from build123d import *

# Parameters (mm, degrees)
SKETCH1_W            = 174
SKETCH1_H            = 65
BOSS_EXTRUDE1_DEPTH  = 5
SKETCH2_W            = 174
SKETCH2_H            = 65
SKETCH2_W_2          = 168
SKETCH2_H_2          = 59
BOSS_EXTRUDE2_DEPTH  = 23
CUT_EXTRUDE2_DEPTH   = 23
SKETCH4_R            = 1.25
CUT_EXTRUDE3_DEPTH   = 4
LPATTERN2_COUNT      = 2
LPATTERN2_PITCH      = 62
LPATTERN2_COUNT_DIR2 = 2
LPATTERN2_PITCH_DIR2 = 171
CUT_EXTRUDE4_DEPTH   = 10


with BuildPart() as part:
    # Sketch1 → Boss-Extrude1 (new body)
    with BuildSketch(Plane(origin=(0, 0, 0), x_dir=(1, 0, 0), z_dir=(0, 1, 0))):
        with Locations((87, 32.5)):
            Rectangle(SKETCH1_W, SKETCH1_H)
    extrude(amount=BOSS_EXTRUDE1_DEPTH)

    # Sketch2 → Boss-Extrude2 (add)
    with BuildSketch(Plane(origin=(0, 5, 0), x_dir=(1, 0, 0), z_dir=(0, 1, 0))):
        with Locations((87, 32.5)):
            Rectangle(SKETCH2_W, SKETCH2_H)
        with Locations((87, 32.5)):
            Rectangle(SKETCH2_W_2, SKETCH2_H_2, mode=Mode.SUBTRACT)
    extrude(amount=BOSS_EXTRUDE2_DEPTH)

    # Sketch3 → Cut-Extrude2 (cut)
    with BuildSketch(Plane(origin=(174, 0, 0), x_dir=(0, 0, -1), z_dir=(1, 0, 0))):
        with BuildLine():
            Line((29.5, 22), (37.5, 22))
            ThreePointArc((37.5, 22), (39.25, 20.25), (37.5, 18.5))
            Line((37.5, 18.5), (29.5, 18.5))
            ThreePointArc((29.5, 18.5), (27.75, 20.25), (29.5, 22))
        make_face()
    extrude(amount=-CUT_EXTRUDE2_DEPTH, mode=Mode.SUBTRACT)

    # Sketch4 → Cut-Extrude3 (cut)
    with BuildSketch(Plane(origin=(0, 28, 0), x_dir=(1, 0, 0), z_dir=(0, 1, 0))):
        with Locations((1.5, 1.5)):
            Circle(SKETCH4_R)
    cut_extrude3 = extrude(amount=-CUT_EXTRUDE3_DEPTH, mode=Mode.SUBTRACT)

    # LPattern2: Cut-Extrude3 2 × 2
    with Locations(*[(j * LPATTERN2_PITCH_DIR2, 0, -i * LPATTERN2_PITCH) for i in range(LPATTERN2_COUNT) for j in range(LPATTERN2_COUNT_DIR2) if (i, j) != (0, 0)]):
        add(cut_extrude3, mode=Mode.SUBTRACT)

    # Sketch5 → Cut-Extrude4 (cut)
    with BuildSketch(Plane.XY):
        with BuildLine():
            Line((128, 15.55), (118, 15.55))
            ThreePointArc((118, 15.55), (115.5, 18.05), (118, 20.55))
            Line((118, 20.55), (128, 20.55))
            ThreePointArc((128, 20.55), (130.5, 18.05), (128, 15.55))
        make_face()
    extrude(amount=-CUT_EXTRUDE4_DEPTH, mode=Mode.SUBTRACT)


solid = part.part
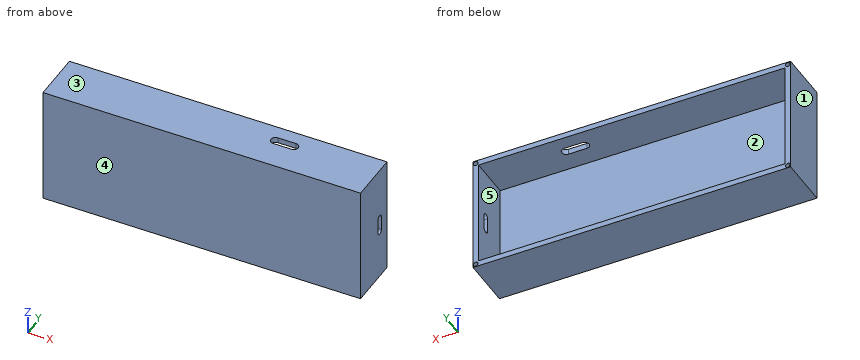
Verification items for the finished model (mm, model axes). Face numbers are marked on the shaded views. A direction names the side the tool comes from. Give positions to 0.01 mm unless a question says otherwise; leave off trailing zeros. Order: outer loops, then holes, each group sorted by start corner. A loop starts at its lowest first (then second) coordinate and runs counter-clockwise, first axis right, second up. Notation, with made-up numbers: M 50,9.25 L 74,9.25 A26 cw 74,24.25 Z; hole C 84,-4.5 d4. An arc over 180 degrees is marked long. Use one line per item in the form item = value. Start each with the question number.
Q1. Go/stop test with flat-tipped pins: pin 1 Ø2 at (x, z) = (172.5, -1.5) entering from +Y; pin 2 Ø1 at (x, z) = (31, -51.5) entering from +Y. Record where each tip stops, or that it passes through.
Q2. Access from +Z, -Z, +X, -X, +Y, -Y to the whole of each face (thin tool, end or side, straight path). Record for the marked faces 1 and 2.
Q3. Section check C-C (z = -51). Enter the section's corners in (x, y).
Q4. Section check B-B (x = 30.5). Enter the section's corners in (y, z).
Q5. Mould release check, pull along Z, two halves, no side actions. Record for the marked faces 3, 4 and 5: +Z half, -Z half, draft (parallel to the pull), parting line (faces both ways), or undercut.
Q6. Scan lines: line 1 along X through (y, z) = (25.45, -63.5); line 2 along Z through (x, y) = (172.5, 25.2); line 3 along Z through (x, y) = (28, 14). Record each from-to range of solid material in increasing order. Write a range as [from, to].
Q7. Section check A-A (y = 11.75). Enter the section's corners in (x, z), then the cut area to 3 significant figures.
Evaluation:
q1.pin_1 = 24
q1.pin_2 = 5
q2.face_1 = +Z, -Z, -X, +Y, -Y
q2.face_2 = +Y
q3.outline = M 0,0 L 174,0 L 174,28 L 171,28 L 171,5 L 3,5 L 3,28 L 0,28 Z
q4.outline = M 0,-65 L 28,-65 L 28,-62 L 5,-62 L 5,-3 L 28,-3 L 28,0 L 0,0 Z
q5.face_3 = +Z half
q5.face_4 = draft
q5.face_5 = undercut
q6.line_1 = [0, 0.25], [2.75, 171.25], [173.75, 174]
q6.line_2 = [-65, -64.75], [-62.25, -2.75], [-0.25, 0]
q6.line_3 = [-65, -62], [-3, 0]
q7.outline = M 0,-65 L 174,-65 L 174,0 L 0,0 Z; hole M 3,-62 L 171,-62 L 171,-3 L 3,-3 Z
q7.area = 1,400 mm2
